Source: CAD feature listing. Evaluate the final solid. Frame: model axes, mm. Round coordinates to 2 decimals unless told otherwise and drop trailing zeros. Order: outer loops, then holes, each group sorted by start corner. A loop starts at its lowest first (then second) coordinate and runs counter-clockwise, first axis right, second up. Notation, with made-up numbers: M 81,66 L 108,66 A8 ccw 108,77 Z; hole C 22,38 d11. An arc over 180 degrees is marked long. Use one line per item in the form item = value. Start each with the question number.
Q1. Material intervals for probe 1 along Y at (x, z) = (50, 2.15); probe 2 along X at (y, z) = (169, 1.6); probe 3 along Y at (x, z) = (44.5, 2.35), sorted ascending.
Q2. Section C-C (x = 47). Return the cut outline in (y, z).
Q3. Section A-A (z = 2.2). Return the cut outline in (x, y), plus the area to 3 significant figures.
Q4. Section B-B (y = 43). Return the cut outline in (x, z), plus the area to 3 significant figures.
Q5. Contact query for flat-ended pins moving along their axis: pin 1 (1.5 mm diameter, centred on y = 26.5, z = 1.5, fed in from +X); pin 2 (1.5 mm diameter, centred on x = 71, z = 0.5, fed in from +Y); pin 3 (1.5 mm diameter, centred on x = 87, z = 1.5, fed in from -Y). Output: stop coordinate, or through.
from build123d import *

# Parameters (mm, degrees)
EXTRUDE_1_DEPTH = 3


with BuildPart() as part:
    # Эскиз1 → Бобышка-Вытянуть1 (new body)
    with BuildSketch(Plane.XY):
        with BuildLine():
            ThreePointArc((71.910596806, 25.230232233), (89.617789367, 131.826316673), (79.68159846, 239.425303641))
            Line((79.68159846, 239.425303641), (32.429608738, 209.371194648))
            ThreePointArc((32.429608738, 209.371194648), (31.080732298, 102.87778502), (-3.3, 2.07782962))
            ThreePointArc((-3.3, 2.07782962), (-1.782749379, 0.828082821), (0, 0))
            Line((0, 0), (71.910596806, 25.230232233))
        make_face()
        with BuildLine():
            ThreePointArc((-3.3, 2.07782962), (31.080732298, 102.87778502), (32.429608738, 209.371194648))
            ThreePointArc((32.429608738, 209.371194648), (30.180601525, 203.45537675), (29.429608738, 197.171194648))
            ThreePointArc((29.429608738, 197.171194648), (23.664975471, 100.000760944), (-5.4, 7.1))
            ThreePointArc((-5.4, 7.1), (-4.805172006, 4.398586498), (-3.3, 2.07782962))
        make_face()
        with BuildLine():
            ThreePointArc((79.68159846, 239.425303641), (88.718866692, 237.000959513), (94.210596806, 229.425303641))
            ThreePointArc((94.210596806, 229.425303641), (102.133781486, 139.336722404), (89.910596806, 49.730232233))
            ThreePointArc((89.910596806, 49.730232233), (81.828404444, 36.80592458), (71.910596806, 25.230232233))
            ThreePointArc((71.910596806, 25.230232233), (89.617789367, 131.826316673), (79.68159846, 239.425303641))
        make_face()
    extrude(amount=EXTRUDE_1_DEPTH)


solid = part.part
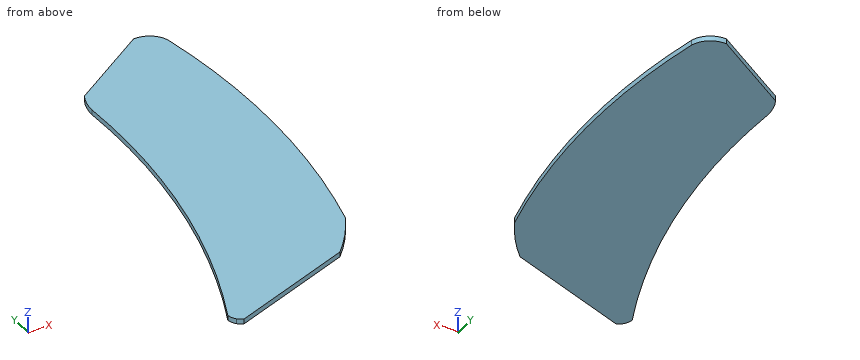
Results list:
q1.probe_1 = 17.54 to 220.55
q1.probe_2 = 30.2 to 101.76
q1.probe_3 = 15.61 to 217.05
q2.outline = M 16.49,0 L 218.64,0 L 218.64,3 L 16.49,3 Z
q3.outline = M -5.4,7.1 A7.75 ccw 0,0 L 71.91,25.23 A102.01 ccw 89.91,49.73 A405.85 ccw 94.21,229.43 A14 ccw 79.68,239.43 L 32.43,209.37 A25.97 ccw 29.43,197.17 A400 cw Z
q3.area = 15,700 mm2
q4.outline = M 8.81,0 L 86.04,0 L 86.04,3 L 8.81,3 Z
q4.area = 232 mm2
q5.pin_1 = 73.87
q5.pin_2 = 234.38
q5.pin_3 = 43.34
